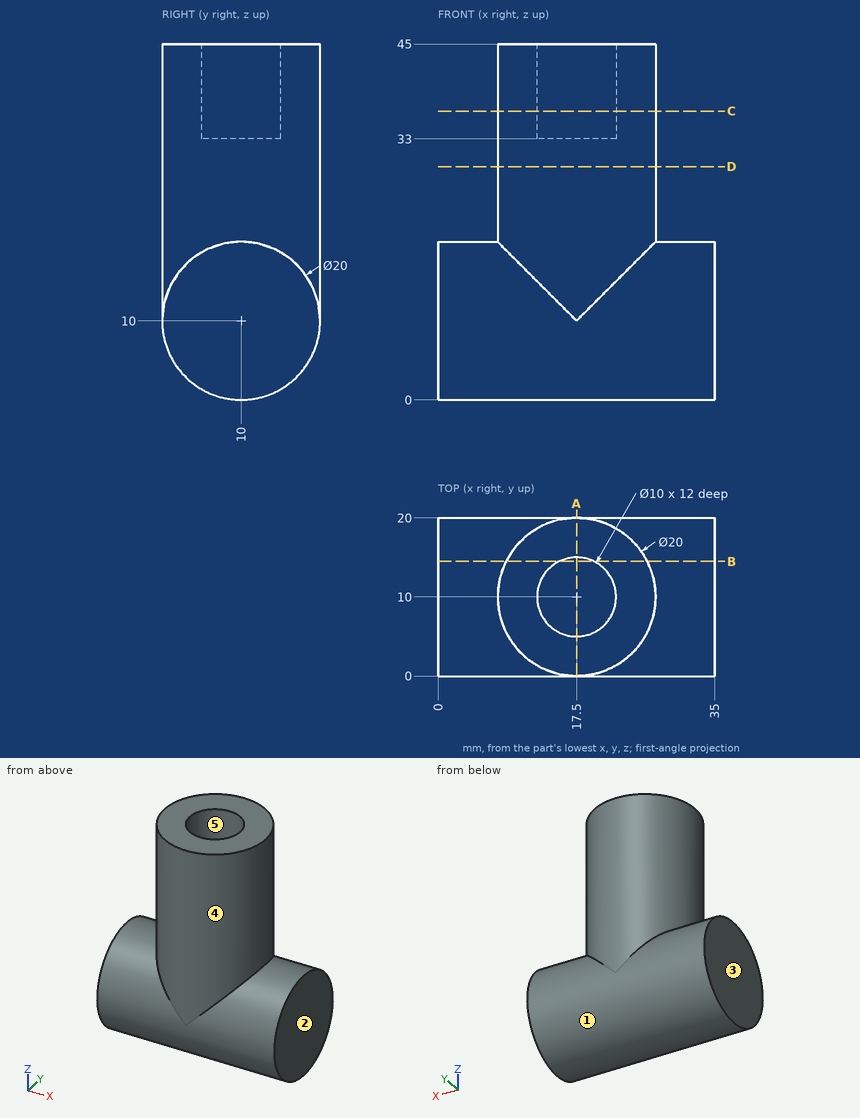
Input: dimensioned drawing with shaded views. Units: mm. Origin: part minimum x, y, z. A direction names the side the tool comes from. Coordinates: 2 decimals unless noted, no trailing zeros. Order: outer loops, then holes, each group sorted by start corner. A loop starts at its lowest first (then second) coordinate and runs counter-clockwise, first axis right, second up.
Item 1: Section query B-B (y = 14.5). Output: boundary loops of the cut face in (x, z).
Answer:
outline: (0, 1.07) - (35, 1.07) - (35, 18.93) - (26.43, 18.93) - (26.43, 45) - (19.68, 45) - (19.68, 33) - (15.32, 33) - (15.32, 45) - (8.57, 45) - (8.57, 18.93) - (0, 18.93) - close
Item 2: Access query for the marked faces 1 and 2. Directions: +Z, -Z, +X, -X, +Y, -Y. A direction counts if a zero-diameter tool reaches every point of the face in a straight line with its end or side. Return the directions, or none.
Answer:
face 1: none
face 2: +Z, -Z, +X, +Y, -Y
Item 3: Section query A-A (x = 17.5). Output: boundary loops of the cut face in (y, z), then the cut area to 3 significant figures.
Answer:
outline: (0, 10) arc R10 ccw to (20, 10) - (20, 45) - (15, 45) - (15, 33) - (5, 33) - (5, 45) - (0, 45) - close
area: 737 mm2
Item 4: Material intervals for line 1 along Y through (x, z) = (17, 42); line 2 along Z through (x, y) = (25, 9.75); line 3 along Z through (x, y) = (3, 17.75), sorted ascending.
Answer:
line 1: y = 0.01 to 5.03, 14.97 to 19.99
line 2: z = 0 to 45
line 3: z = 3.68 to 16.32
Item 5: Contact query for flat-ended pins moving along their axis: P1, Ø3, axis at x = 14, z = 35, coming from the +Y side; P2, Ø6, axis at x = 27, z = 36, coming from the +Y side; P3, Ø4, axis at x = 13.5, y = 15.5, coming from the -Z side. Output: stop coordinate, or through.
Answer:
P1: stops at y = 19.8
P2: stops at y = 17.6
P3: stops at z = 0.63
Item 6: Section query C-C (z = 36.5). Output: boundary loops of the cut face in (x, y).
Answer:
outline: circle Ø20 at (17.5, 10); hole circle Ø10 at (17.5, 10)
Item 7: Section query D-D (z = 29.5). Output: boundary loops of the cut face in (x, y).
Answer:
outline: circle Ø20 at (17.5, 10)
Item 8: Draft query along X for the marked faces 3, 4 and 5. Return one class per face: released by +X, released by -X, zero draft, split by the parting line, or undercut.
Answer:
face 3: released by -X
face 4: split by the parting line
face 5: undercut
